from build123d import *

# Parameters (mm, degrees)
SKETCH2_R           = 8
BOSS_EXTRUDE1_DEPTH = 20
SKETCH3_R           = 10
BOSS_EXTRUDE2_DEPTH = 6
SKETCH1_R           = 4
CUT_EXTRUDE1_DEPTH  = 25.494897428


with BuildPart() as part:
    # Sketch2 → Boss-Extrude1 (new body)
    with BuildSketch(Plane(origin=(0, 0, 0), x_dir=(1, 0, 0), z_dir=(0, 1, 0))):
        with Locations(Location((0, 0, 0), (0, 0, 270))):
            Circle(SKETCH2_R)
    extrude(amount=BOSS_EXTRUDE1_DEPTH)

    # Sketch3 → Boss-Extrude2 (add)
    with BuildSketch(Plane(origin=(0, 0, 0), x_dir=(1, 0, 0), z_dir=(0, 1, 0))):
        with Locations(Location((0, 0, 0), (0, 0, 270))):
            Circle(SKETCH3_R)
    extrude(amount=BOSS_EXTRUDE2_DEPTH)

    # Sketch1 → Cut-Extrude1 (cut, through all)
    with BuildSketch(Plane(origin=(0, 0, 0), x_dir=(1, 0, 0), z_dir=(0, 1, 0))):
        with Locations(Location((0, 0, 0), (0, 0, 270))):
            Circle(SKETCH1_R)
    extrude(amount=CUT_EXTRUDE1_DEPTH, mode=Mode.SUBTRACT)


solid = part.part
For this review, take the finished solid that the model builds, in its own axes (mm). A direction names the side the tool comes from. Round coordinates to 2 decimals unless told otherwise and drop trailing zeros. Write each loop counter-clockwise with the first axis right and the second up, starting at its lowest first coordinate (ties: lowest second). Pieces come first, ordered by that corner, then holes. Notation, with made-up numbers: (-29, 80.5) - (25, 80.5) arc R27 ccw to (25, 101.5) - close; hole circle Ø3 at (3, 48). An arc over 180 degrees is marked (long way). Use a Markdown table: item, result.
Q1. We need section A-A (z = 0). Give the boundary of the cut face in (x, y).
Derived:
| item | result |
|---|---|
| outline | (-10, 0) - (-4, 0) - (-4, 20) - (-8, 20) - (-8, 6) - (-10, 6) - close; (4, 0) - (10, 0) - (10, 6) - (8, 6) - (8, 20) - (4, 20) - close |
Q2. We need section D-D (x = -5). Give the boundary of the cut face in (y, z) (3 decimals), plus the area to 3 significant figures.
Derived:
| item | result |
|---|---|
| outline | (0, -8.66) - (6, -8.66) - (6, -6.245) - (20, -6.245) - (20, 6.245) - (6, 6.245) - (6, 8.66) - (0, 8.66) - close |
| area | 279 mm2 |
Q3. Clearance check with flat-ended pins moving along their axes: pin 1 (1 mm diameter, centred on x = -0.5, y = 17, fed in from +Z); pin 2 (4 mm diameter, centred on y = 17.5, z = -7.5, fed in from -X); pin 3 (5 mm diameter, centred on x = 0, z = 0, fed in from +Y); pin 4 (3 mm diameter, centred on y = 15.5, z = -4, fed in from -X). State where each tip first meets the part, or that it passes through.
Derived:
| item | result |
|---|---|
| pin 1 | stops at z = 8 |
| pin 2 | stops at x = -5.81 |
| pin 3 | passes through |
| pin 4 | stops at x = -7.6 |
Q4. We need section C-C (y = 4.5). Give the boundary of the cut face in (x, z).
Derived:
| item | result |
|---|---|
| outline | circle Ø20 at (0, 0); hole circle Ø8 at (0, 0) |
Q5. The part is to be moulded in two halves that separate along Z. For faces 1 (the cylindrical face through (-9.76, 2.96, -2.17)), 2 (the cylindrical face through (-3.905, 9.86, -0.867)), 3 (the flat face through (8.2, 6, 0)), say which applies: pulls with the +Z half, pulls with the -Z half, needs draft (parallel to the pull), parting line crosses it, or undercut.
Derived:
| item | result |
|---|---|
| face 1 | parting line crosses it |
| face 2 | undercut |
| face 3 | needs draft |
Q6. Machinability: for faces 4 (the flat face through (0.1, 0, 4.3)), 5 (the cylindrical face through (-7.81, 12.9, -1.73)), which of the approach directions +Z, -Z, +X, -X, +Y, -Y give a long, thin tool a straight path to every point of the face, cutting with its end or side? Answer none if there is none.
Derived:
| item | result |
|---|---|
| face 4 | +Z, -Z, +X, -X, -Y |
| face 5 | +Y |
Q7. We need section B-B (x = 0). Give the boundary of the cut face in (y, z).
Derived:
| item | result |
|---|---|
| outline | (0, -10) - (6, -10) - (6, -8) - (20, -8) - (20, -4) - (0, -4) - close; (0, 4) - (20, 4) - (20, 8) - (6, 8) - (6, 10) - (0, 10) - close |
Q8. Wall thickness on line 1 along Z through (x, y) = (0, 10.5); line 2 along Y through (x, z) = (5.5, 8): over which ranges is each line inside the solid? List them lowest first.
Derived:
| item | result |
|---|---|
| line 1 | z = -8 to -4, 4 to 8 |
| line 2 | y = 0 to 6 |
